Source: three-view drawing plus pictorial views. Frame: mm from the lowest corner of the part. A direction names the side the tool comes from. Give positions to 0.01 mm unless a question says otherwise; leave off trailing zeros. Loops run counter-clockwise (first coordinate to the right, second up) from the corner with the lowest first, then second, coordinate; pieces in that order, holes last. Notation, with made-up numbers: M 23.5,32.25 L 73.5,32.25 A16 cw 73.5,49.25 Z; hole C 69.5,74.25 d1. An arc over 180 degrees is marked long. Write item = value, one per line.
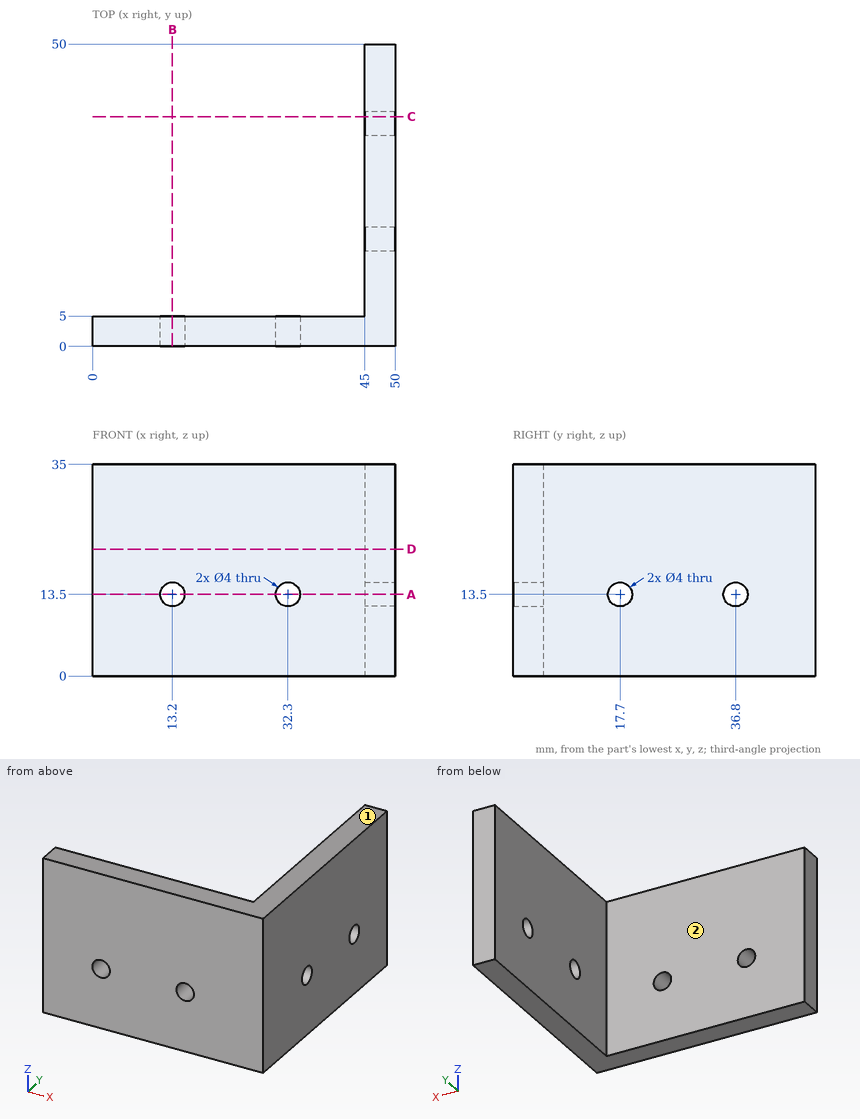
1. Material intervals for probe 1 along X at (y, z) = (2.75, 13.5); probe 2 along Y at (x, z) = (48, 13); probe 3 along Z at (x, y) = (13.2, 1.7), sorted ascending. Write a range as from..to.
Derived:
probe_1 = 0..11.2, 15.2..30.3, 34.3..50
probe_2 = 0..15.76, 19.64..34.86, 38.74..50
probe_3 = 0..11.5, 15.5..35
2. Cut plane A-A, the plane z = 13.5. Return the cut outline in (x, y), then the cut area to 3 significant figures.
Derived:
outline = M 0,0 L 11.2,0 L 11.2,5 L 0,5 Z; M 15.2,0 L 30.3,0 L 30.3,5 L 15.2,5 Z; M 34.3,0 L 50,0 L 50,15.7 L 45,15.7 L 45,5 L 34.3,5 Z; M 45,19.7 L 50,19.7 L 50,34.8 L 45,34.8 Z; M 45,38.8 L 50,38.8 L 50,50 L 45,50 Z
area = 395 mm²
3. First-contact query: pin 1 Ø5 at (x, z) = (32.3, 13.5) entering from +Y; pin 2 Ø5 at (y, z) = (17.7, 13.5) entering from +X; pin 3 Ø5 at (y, z) = (36.8, 13.5) entering from -X. Flat tips, straight axial feed; report the tip coordinate or a pass-through.
Derived:
pin_1 = 5
pin_2 = 50
pin_3 = 45
4. Cut plane B-B, the plane x = 13.2. Return the cut outline in (y, z).
Derived:
outline = M 0,0 L 5,0 L 5,11.5 L 0,11.5 Z; M 0,15.5 L 5,15.5 L 5,35 L 0,35 Z
5. Cut plane D-D, the plane z = 21. Return the cut outline in (x, y).
Derived:
outline = M 0,0 L 50,0 L 50,50 L 45,50 L 45,5 L 0,5 Z
6. Reachability of the marked faces 1 and 2 from +Z, -Z, +X, -X, +Y, -Y: full face, straight path, thin tool, end or side. Return the list, or none.
Derived:
face_1 = +Z, +X, -X, +Y, -Y
face_2 = +Z, -Z, -X, +Y
7. Cut plane C-C, the plane y = 38. Return the cut outline in (x, z).
Derived:
outline = M 45,0 L 50,0 L 50,11.9 L 45,11.9 Z; M 45,15.1 L 50,15.1 L 50,35 L 45,35 Z
